Check sheet for the modelled part. Datum: model origin and axes. Units: mm. A direction names the side the tool comes from. Give positions to 0.01 mm unless a question says otherwise; leave off trailing zeros. Loops run counter-clockwise (first coordinate to the right, second up) from the corner with the lowest first, then second, coordinate; pieces in that order, holes last. Notation, with made-up numbers: (59, 50) - (88, 50) arc R27 cw to (88, 85) - close; hole circle Ø11 at (68.25, -7.5). An arc over 180 degrees is marked (long way). Use one line per item in the form item = value.
from build123d import *

# Parameters (mm, degrees)
BOSS_EXTRUDE1_DEPTH = 2
SKETCH3_R           = 3.5
SKETCH3_R_2         = 2.5
BOSS_EXTRUDE2_DEPTH = 6
SKETCH4_R           = 1.25
CUT_EXTRUDE1_DEPTH  = 1
SKETCH5_R           = 0.5
CUT_EXTRUDE2_DEPTH  = 15.525839337


with BuildPart() as part:
    # Sketch2 → Boss-Extrude1 (new body)
    with BuildSketch(Plane.XY):
        with BuildLine():
            Line((1.49, -7.68), (2.28, -4.48))
            ThreePointArc((2.28, -4.48), (2.535701974, -3.719084235), (3.07, -3.12))
            ThreePointArc((3.07, -3.12), (3.084239628, -3.109259088), (3.098353652, -3.098353652))
            ThreePointArc((3.098353652, -3.098353652), (3.109259088, -3.084239628), (3.12, -3.07))
            ThreePointArc((3.12, -3.07), (3.719084235, -2.535701974), (4.48, -2.28))
            Line((4.48, -2.28), (7.68, -1.49))
            ThreePointArc((7.68, -1.49), (8.622775638, -0.995512646), (9, 0))
            ThreePointArc((9, 0), (8.622775638, 0.995512646), (7.68, 1.49))
            Line((7.68, 1.49), (4.48, 2.28))
            ThreePointArc((4.48, 2.28), (3.719084235, 2.535701974), (3.12, 3.07))
            ThreePointArc((3.12, 3.07), (3.109259088, 3.084239628), (3.098353652, 3.098353652))
            ThreePointArc((3.098353652, 3.098353652), (3.084239628, 3.109259088), (3.07, 3.12))
            ThreePointArc((3.07, 3.12), (2.535701974, 3.719084235), (2.28, 4.48))
            Line((2.28, 4.48), (1.49, 7.68))
            ThreePointArc((1.49, 7.68), (0.995512646, 8.622775638), (0, 9))
            ThreePointArc((0, 9), (-0.995512646, 8.622775638), (-1.49, 7.68))
            Line((-1.49, 7.68), (-2.28, 4.48))
            ThreePointArc((-2.28, 4.48), (-2.535701974, 3.719084235), (-3.07, 3.12))
            ThreePointArc((-3.07, 3.12), (-3.084239628, 3.109259088), (-3.098353652, 3.098353652))
            ThreePointArc((-3.098353652, 3.098353652), (-3.109259088, 3.084239628), (-3.12, 3.07))
            ThreePointArc((-3.12, 3.07), (-3.719084235, 2.535701974), (-4.48, 2.28))
            Line((-4.48, 2.28), (-7.68, 1.49))
            ThreePointArc((-7.68, 1.49), (-8.622775638, 0.995512646), (-9, 0))
            ThreePointArc((-9, 0), (-8.622775638, -0.995512646), (-7.68, -1.49))
            Line((-7.68, -1.49), (-4.48, -2.28))
            ThreePointArc((-4.48, -2.28), (-3.719084235, -2.535701974), (-3.12, -3.07))
            ThreePointArc((-3.12, -3.07), (-3.109259088, -3.084239628), (-3.098353652, -3.098353652))
            ThreePointArc((-3.098353652, -3.098353652), (-3.084239628, -3.109259088), (-3.07, -3.12))
            ThreePointArc((-3.07, -3.12), (-2.535701974, -3.719084235), (-2.28, -4.48))
            Line((-2.28, -4.48), (-1.49, -7.68))
            ThreePointArc((-1.49, -7.68), (-0.995512646, -8.622775638), (0, -9))
            ThreePointArc((0, -9), (0.995512646, -8.622775638), (1.49, -7.68))
        make_face()
    extrude(amount=BOSS_EXTRUDE1_DEPTH)

    # Sketch3 → Boss-Extrude2 (add)
    with BuildSketch(Plane.XY.offset(2)):
        Circle(SKETCH3_R)
        Circle(SKETCH3_R_2, mode=Mode.SUBTRACT)
    extrude(amount=BOSS_EXTRUDE2_DEPTH)

    # Sketch4 → Cut-Extrude1 (cut)
    with BuildSketch(Plane(origin=(0, 0, 0), x_dir=(-1, 0, 0), z_dir=(0, 0, -1))):
        Circle(SKETCH4_R)
    extrude(amount=-CUT_EXTRUDE1_DEPTH, mode=Mode.SUBTRACT)

    # Sketch5 → Cut-Extrude2 (cut, through all)
    with BuildSketch(Plane(origin=(0, 0, 1), x_dir=(-1, 0, 0), z_dir=(0, 0, -1))):
        Circle(SKETCH5_R)
    extrude(amount=-CUT_EXTRUDE2_DEPTH, mode=Mode.SUBTRACT)


solid = part.part
Item 1: Mould release check, pull along Y, two halves, no side actions. Record for faces 1 (the face through (0.27, -1.22, 0.49)), 2 (the face through (2, 0, 0)), 3 (the face through (6.1, 1.88, 0.99)): released by +Y, released by -Y, zero draft, split by the parting line, or undercut.
Answer block:
face_1 = undercut
face_2 = zero draft
face_3 = released by +Y
Item 2: Gauge pin test, flat ends, axial feed: P1, Ø5, axis at x = 5.5, y = 3, coming from the +Z side; P2, Ø6.5, axis at x = 0, y = 0, coming from the +Z side; P3, Ø1, axis at y = 6.5, z = 3.5, coming from the -X side; P4, Ø1.5, axis at y = -1, z = 1, coming from the +X side. Record the tip position at first contact, or that the pin passes through.
Answer block:
P1 = 2
P2 = 8
P3 = through
P4 = 8.98
Item 3: Section check B-B on y = -2.75. Record the boundary of the cut face in (x, z).
Answer block:
outline = (-3.42, 0) - (3.42, 0) - (3.42, 2) - (2.17, 2) - (2.17, 8) - (-2.17, 8) - (-2.17, 2) - (-3.42, 2) - close
Item 4: Access from +Z, -Z, +X, -X, +Y, -Y to the whole of each face (thin tool, end or side, straight path). Record for faces 4 (the face through (1.88, -6.1, 0.99)), 5 (the face through (-1.4, 3.4, 2)).
Answer block:
face_4 = +Z, -Z, +X, -Y
face_5 = +Z
Item 5: Section check D-D on z = 6. Record the boundary of the cut face in (x, y), then the cut area to 3 significant figures.
Answer block:
outline = circle Ø7 at (0, 0); hole circle Ø5 at (0, 0)
area = 18.8 mm2
Item 6: Section check C-C on x = 6. Record the boundary of the cut face in (y, z).
Answer block:
outline = (-1.9, 0) - (1.9, 0) - (1.9, 2) - (-1.9, 2) - close
Item 7: Thickness scan on L1, parallel to Y at x = 0, z = 3.3; L2, parallel to Y at x = -4.5, z = 0.75; L3, parallel to Z at x = 0.75, y = 4. Record the ranges inside material, lowest first.
Answer block:
L1 = -3.5 to -2.5, 2.5 to 3.5
L2 = -2.28 to 2.28
L3 = 0 to 2
